CAD build for the part. Positions are in the model's coordinates, mm. Face numbers are marked on the shaded views. A direction names the side the tool comes from. Give positions to 0.01 mm unless a question says otherwise; leave off trailing zeros. Order: outer loops, then holes, each group sorted by start corner. A loop starts at its lowest first (then second) coordinate and runs counter-clockwise, first axis right, second up.
Item 1: Wall check: L1, parallel to X at y = 502, z = 17.5; L2, parallel to Y at x = -472.5, z = 15.5; L3, parallel to Y at x = -2, z = -8.5. Give the ranges that are in metal, low to high.
Item 2: Band-saw the part on A-A on z = 1. Give the cut face in (x, y), plus the area to 3 significant figures.
Item 3: Which spindle directions (+Z, -Z, +X, -X, +Y, -Y) get a long thin tool onto all of the face, cutting with end or side? Do the marked faces 1 and 2. Say none if no direction does.
Item 4: Band-saw the part on C-C on x = -230.5. Give the cut face in (y, z), plus the area to 3 significant figures.
Item 5: Band-saw the part on B-B on y = 543.5. Give the cut face in (x, z), plus the area to 3 significant figures.
Item 6: Flat gauge pins, fed straight in: P1, Ø2, axis at y = 61.5, z = -16.5, coming from the -X side; P2, Ø6, axis at x = -85, z = -12, coming from the -Y side. Where does each tip first touch, or does it go through?
```python
from build123d import *

# Parameters (mm, degrees)
F1_W   = 50.8
F1_H   = 50.8
F1_W_2 = 38.1
F1_H_2 = 38.1


with BuildPart() as f2:
    # F2: sweep along a path in F0
    with BuildLine(Plane.XY) as f2_path:
        Line((0, 0), (0, 584.2))
        Line((0, 584.2), (-584.2, 584.2))
    # F1 (on Front) → F2 (sweep)
    with BuildSketch(Plane.XZ):
        Rectangle(F1_W, F1_H)
        Rectangle(F1_W_2, F1_H_2, mode=Mode.SUBTRACT)
    sweep(path=f2_path.line, transition=Transition.RIGHT)


solid = f2.part
```
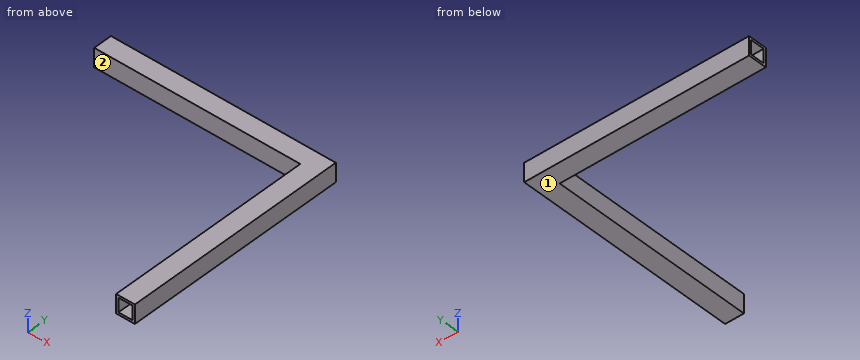
The answers:
1. L1: x = -25.4 to -19.05, 19.05 to 25.4
1. L2: y = 558.8 to 565.15, 603.25 to 609.6
1. L3: y = 603.25 to 609.6
2. outline: (-584.2, 558.8) - (-25.4, 558.8) - (-25.4, 0) - (-19.05, 0) - (-19.05, 565.15) - (-584.2, 565.15) - close; (-584.2, 603.25) - (19.05, 603.25) - (19.05, 0) - (25.4, 0) - (25.4, 609.6) - (-584.2, 609.6) - close
2. area: 14,800 mm2
3. face 1: -Z, +X, -X, +Y, -Y
3. face 2: +Z, -Z, -X, -Y
4. outline: (558.8, -25.4) - (609.6, -25.4) - (609.6, 25.4) - (558.8, 25.4) - close; hole (565.15, -19.05) - (603.25, -19.05) - (603.25, 19.05) - (565.15, 19.05) - close
4. area: 1,130 mm2
5. outline: (-25.4, -25.4) - (25.4, -25.4) - (25.4, 25.4) - (-25.4, 25.4) - close; hole (-19.05, -19.05) - (19.05, -19.05) - (19.05, 19.05) - (-19.05, 19.05) - close
5. area: 1,130 mm2
6. P1: stops at x = -25.4
6. P2: stops at y = 558.8
